from build123d import *

# Parameters (mm, degrees)
SKETCH1_R           = 1.65
BOSS_EXTRUDE1_DEPTH = 4.5


with BuildPart() as part:
    # Sketch1 → Boss-Extrude1 (new body)
    with BuildSketch(Plane(origin=(0, 0, 0), x_dir=(1, 0, 0), z_dir=(0, 1, 0))):
        with BuildLine():
            Line((6.25, 6.25), (6.25, 0))
            ThreePointArc((6.25, 0), (0, -6.25), (-6.25, 0))
            Line((-6.25, 0), (-6.25, 6.25))
            ThreePointArc((-6.25, 6.25), (-9.179700773, 10.519130601), (-14.216868268, 9.320979382))
            ThreePointArc((-14.216868268, 9.320979382), (-14.722431864, 8.5), (-15.180639067, 7.651679391))
            ThreePointArc((-15.180639067, 7.651679391), (0, -17), (15.180639067, 7.651679391))
            ThreePointArc((15.180639067, 7.651679391), (14.722431864, 8.5), (14.216868268, 9.320979382))
            ThreePointArc((14.216868268, 9.320979382), (9.179700773, 10.519130601), (6.25, 6.25))
        make_face()
        with Locations((-10.825317547, -6.25)):
            Circle(SKETCH1_R, mode=Mode.SUBTRACT)
        with Locations((0, -12.5)):
            Circle(SKETCH1_R, mode=Mode.SUBTRACT)
        with Locations((10.825317547, -6.25)):
            Circle(SKETCH1_R, mode=Mode.SUBTRACT)
        with Locations((-10.825317547, 6.25)):
            Circle(SKETCH1_R, mode=Mode.SUBTRACT)
        with Locations((10.825317547, 6.25)):
            Circle(SKETCH1_R, mode=Mode.SUBTRACT)
    extrude(amount=BOSS_EXTRUDE1_DEPTH)


solid = part.part
Part model, mm, in its own coordinate system. A direction names the side the tool comes from. Coordinates: 2 decimals unless noted, no trailing zeros. Loops run counter-clockwise (first coordinate to the right, second up) from the corner with the lowest first, then second, coordinate; pieces in that order, holes last. Notation, with made-up numbers: (-0.75, -10) - (7.25, -10) arc R31 ccw to (7.25, 25) - close; hole circle Ø9 at (73, 82.25). An arc over 180 degrees is marked (long way). Write each question's results on one line, items separated by ' | '. Start each with the question number.
Q1. Slice it at C-C on x = 0. Give the cut face in (y, z).
Q2. Slice it at A-A on y = 2.55. Give the cut face in (x, z).
Q3. Drop flat-ended pins along their axis: pin 1 Ø3 at (x, z) = (0, 12.5) entering from +Y; pin 2 Ø2 at (y, z) = (3, 2.5) entering from -X; pin 3 Ø2 at (y, z) = (2.5, -2) entering from -X. Give the stop position or say it passes through.
Q4. Which spindle directions (+Z, -Z, +X, -X, +Y, -Y) get a long thin tool onto all of the face, cutting with end or side? Do faces 3 (the flat face through (6.25, 2, -3)), 4 (the flat face through (-4, 4.5, 6)). Say none if no direction does.
Q5. Slice it at D-D on x = 12. Give the cut face in (y, z), and give its area (3 significant figures).
Q6. Probe line 1 along Z through (x, y) = (0, 2.5); line 2 along X through (y, z) = (2.45, -5.25); line 3 along X through (y, z) = (2, -6.75). List the from-to ranges inside material, lowest first.
Q7. Slice it at B-B on z = 6.75. Give the cut face in (x, y).
Q8. Two-plate mould, pull along X, no slides. Class faces 1 (the cylindrical face through (-0.4, 2.2, 14.1)), 2 (the flat face through (-4, 0, 6)): +X half, -X half, draft (parallel to the pull), parting line (faces both ways), or undercut.
Answer:
1) outline: (0, 6.25) - (4.5, 6.25) - (4.5, 10.85) - (0, 10.85) - close; (0, 14.15) - (4.5, 14.15) - (4.5, 17) - (0, 17) - close
2) outline: (-14.22, -9.32) arc R4.58 ccw to (-6.25, -6.25) - (-6.25, 0) arc R6.25 cw to (6.25, 0) - (6.25, -6.25) arc R4.58 ccw to (14.22, -9.32) arc R17 ccw (long way) to start; hole circle Ø3.3 at (-10.83, -6.25); hole circle Ø3.3 at (-10.83, 6.25); hole circle Ø3.3 at (0, 12.5); hole circle Ø3.3 at (10.83, -6.25); hole circle Ø3.3 at (10.83, 6.25)
3) pin 1: passes through | pin 2: stops at x = -16.93 | pin 3: stops at x = -16.97
4) face 3: -Z, +Y, -Y | face 4: +Z, -Z, +X, -X, +Y
5) outline: (0, -10.67) - (4.5, -10.67) - (4.5, -7.41) - (0, -7.41) - close; (0, -5.09) - (4.5, -5.09) - (4.5, 5.09) - (0, 5.09) - close; (0, 7.41) - (4.5, 7.41) - (4.5, 12.04) - (0, 12.04) - close | area: 81.4 mm2
6) line 1: z = 6.25 to 10.85, 14.15 to 17 | line 2: x = -16.17 to -12.14, -9.51 to -6.25, 6.25 to 9.51, 12.14 to 16.17 | line 3: x = -15.6 to -12.4, -9.25 to -6.28, 6.28 to 9.25, 12.4 to 15.6
7) outline: (-15.6, 0) - (-12.4, 0) - (-12.4, 4.5) - (-15.6, 4.5) - close; (-9.25, 0) - (9.25, 0) - (9.25, 4.5) - (-9.25, 4.5) - close; (12.4, 0) - (15.6, 0) - (15.6, 4.5) - (12.4, 4.5) - close
8) face 1: undercut | face 2: draft
